Work out the finished part from the listing and answer in its coordinate system (mm). A direction names the side the tool comes from. Coordinates: 2 decimals unless noted, no trailing zeros. Order: outer loops, then holes, each group sorted by start corner. A loop starts at its lowest first (then second) coordinate and runs counter-clockwise, first axis right, second up. Notation, with made-up numbers: M 58,65.25 L 91,65.25 A22 cw 91,82.25 Z; hole C 23,-15.75 d3. An arc over 180 degrees is marked long. Answer in a Markdown table with one row per item. Add a question column.
Item 1: The part is cut by section C-C (y = -1.25). Write down the section's boundary in (x, z), then the cut area to 3 significant figures.
Item 2: Consider line 1 (X direction, y = -9.75, z = 37); line 2 (Y direction, x = 0, z = 9); line 3 (Z direction, x = -2.5, y = -8.5). Determine where each line is inside the solid, lowest interval first. Write a range as from..to.
Item 3: The part is cut by section A-A (y = -10.25). Write down the section's boundary in (x, z).
Item 4: The mould has two halves that part along Y. Classify faces 1 (the face through (10, -4, 38)), 2 (the face through (-1.46, -6.59, 20.28)), 3 (the face through (0, -12, 37)), 4 (the face through (13.6, -7, 1.6)): released by +Y, released by -Y, zero draft, split by the parting line, or undercut.
Item 5: Flat-ended cylindrical pins translate along their axes: pin 1 Ø1.5 at (x, y) = (12, -2.5) entering from +Z; pin 2 Ø10 at (x, y) = (12.5, 5) entering from -Z; pin 3 Ø8 at (y, z) = (4.5, 27) entering from -X; pin 4 Ø6.5 at (x, z) = (-11, 36) entering from +Y. Find the tip coordinate at first contact, or state that the pin passes through.
Item 6: The part is cut by section D-D (z = 24). Write down the section's boundary in (x, y).
Item 7: Which of the six approach directions +Z, -Z, +X, -X, +Y, -Y give full straight-line access (tool end or side, diameter ignored) to faces 5 (the face through (-11, -3, 35)), 6 (the face through (-10, -3, 2)), 7 (the face through (10, -4, 2)), 8 (the face through (11, -4, 4))?
Item 8: The part is cut by section B-B (x = -15). Write down the section's boundary in (y, z).
from build123d import *

# Parameters (mm, degrees)
BOSS_EXTRUDE1_DEPTH = 6
SKETCH2_R           = 7.5
BOSS_EXTRUDE2_DEPTH = 28
BOSS_EXTRUDE3_DEPTH = 6
SKETCH4_R           = 6.75
CUT_EXTRUDE1_DEPTH  = 46.880278988
SKETCH6_R           = 1.75
CUT_EXTRUDE3_DEPTH  = 48.801673611
CHAMFER1_SIZE       = 3


with BuildPart() as part:
    # Sketch1 → Boss-Extrude1 (new body)
    with BuildSketch(Plane.XY):
        with BuildLine():
            Line((-11, 0), (-11, -7))
            Line((-11, -7), (-19, -7))
            Line((-19, -7), (-19, -12))
            Line((-19, -12), (-11, -12))
            Line((-11, -12), (11, -12))
            Line((11, -12), (19, -12))
            Line((19, -12), (19, -7))
            Line((19, -7), (11, -7))
            Line((11, -7), (11, 0))
            ThreePointArc((11, 0), (0, 11), (-11, 0))
        make_face()
    extrude(amount=BOSS_EXTRUDE1_DEPTH)

    # Sketch2 → Boss-Extrude2 (add)
    with BuildSketch(Plane.XY.offset(6)):
        Circle(SKETCH2_R)
    extrude(amount=BOSS_EXTRUDE2_DEPTH)

    # Sketch3 → Boss-Extrude3 (add)
    with BuildSketch(Plane.XY.offset(34)):
        with BuildLine():
            Line((-11, 0), (-11, -7))
            Line((-11, -7), (-19, -7))
            Line((-19, -7), (-19, -12))
            Line((-19, -12), (19, -12))
            Line((19, -12), (19, -7))
            Line((19, -7), (11, -7))
            Line((11, -7), (11, 0))
            ThreePointArc((11, 0), (0, 11), (-11, 0))
        make_face()
    extrude(amount=BOSS_EXTRUDE3_DEPTH)

    # Sketch4 → Cut-Extrude1 (cut, through all)
    with BuildSketch(Plane.XY.offset(40)):
        Circle(SKETCH4_R)
    extrude(amount=-CUT_EXTRUDE1_DEPTH, mode=Mode.SUBTRACT)

    # Sketch6 → Cut-Extrude3 (cut, through all)
    with BuildSketch(Plane(origin=(0, -7, 0), x_dir=(1, 0, 0), z_dir=(0, 1, 0))):
        with Locations(Location((-15, -3, 0), (0, 0, 270))):
            Circle(SKETCH6_R)
        with Locations(Location((15, -3, 0), (0, 0, 270))):
            Circle(SKETCH6_R)
        with Locations(Location((15, -37, 0), (0, 0, 270))):
            Circle(SKETCH6_R)
        with Locations(Location((-15, -37, 0), (0, 0, 270))):
            Circle(SKETCH6_R)
    extrude(amount=-CUT_EXTRUDE3_DEPTH, mode=Mode.SUBTRACT)

    # Chamfer1
    chamfer1_edges = [part.edges().sort_by_distance(p)[0] for p in [
        (-11, -3.5, 0),
        (0, 11, 0),
        (11, -3.5, 0),
        (11, -3.5, 40),
        (0, 11, 40),
        (-11, -3.5, 40),
    ]]
    chamfer(chamfer1_edges, length=CHAMFER1_SIZE)


solid = part.part
Reply:
| question | item | result |
|---|---|---|
| 1 | outline | M -11,3 L -8,0 L -6.63,0 L -6.63,40 L -8,40 L -11,37 L -11,34 L -7.4,34 L -7.4,6 L -11,6 Z; M 6.63,0 L 8,0 L 11,3 L 11,6 L 7.4,6 L 7.4,34 L 11,34 L 11,37 L 8,40 L 6.63,40 Z |
| 1 | area | 129 mm2 |
| 2 | line 1 | x = -19..-16.75, -13.25..13.25, 16.75..19 |
| 2 | line 2 | y = -7.5..-6.75, 6.75..7.5 |
| 2 | line 3 | z = 0..6, 34..40 |
| 3 | outline | M -19,0 L 19,0 L 19,6 L -19,6 Z; M -19,34 L 19,34 L 19,40 L -19,40 Z; hole C -15,3 d3.5; hole C -15,37 d3.5; hole C 15,3 d3.5; hole C 15,37 d3.5 |
| 4 | face 1 | zero draft |
| 4 | face 2 | undercut |
| 4 | face 3 | released by -Y |
| 4 | face 4 | released by +Y |
| 5 | pin 1 | passes through |
| 5 | pin 2 | stops at z = 0.46 |
| 5 | pin 3 | stops at x = -7.48 |
| 5 | pin 4 | stops at y = 7.81 |
| 6 | outline | C 0,0 d15; hole C 0,0 d13.5 |
| 7 | face 5 | +Z, -Z, -X, +Y |
| 7 | face 6 | -Z, -X, +Y |
| 7 | face 7 | -Z, +X, +Y |
| 7 | face 8 | +Z, -Z, +X, +Y |
| 8 | outline | M -12,0 L -7,0 L -7,1.25 L -12,1.25 Z; M -12,4.75 L -7,4.75 L -7,6 L -12,6 Z; M -12,34 L -7,34 L -7,35.25 L -12,35.25 Z; M -12,38.75 L -7,38.75 L -7,40 L -12,40 Z |
